from build123d import *

# Parameters (mm, degrees)
EXTRUDE_START   = 0.25
SKETCH_1_R      = 1.7
EXTRUDE_1_DEPTH = 6.5
SKETCH_2_R      = 5
SKETCH_2_R_2    = 1.7
EXTRUDE_2_DEPTH = 3


with BuildPart() as part:
    # 草图1 → 凸台-拉伸1 (new body)
    with BuildSketch(Plane.XY.offset(EXTRUDE_START)):
        with BuildLine():
            Line((198.226260921, 33.007621373), (206.908669804, -16.232766278))
            ThreePointArc((206.908669804, -16.232766278), (205.255667217, -20.882583864), (200.416253934, -21.848658507))
            Line((200.416253934, -21.848658507), (152.961109764, -6.171946743))
            ThreePointArc((152.961109764, -6.171946743), (148.598749605, -1.128713155), (150.97313978, 5.10239128))
            Line((150.97313978, 5.10239128), (190.204637372, 36.064296853))
            ThreePointArc((190.204637372, 36.064296853), (195.08261531, 36.811660465), (198.226260921, 33.007621373))
        make_face()
        with Locations((201.984631039, -17.101007166)):
            Circle(SKETCH_1_R, mode=Mode.SUBTRACT)
        with Locations((155, 0)):
            Circle(SKETCH_1_R, mode=Mode.SUBTRACT)
        with Locations((193.302222156, 32.139380484)):
            Circle(SKETCH_1_R, mode=Mode.SUBTRACT)
    extrude(amount=EXTRUDE_1_DEPTH)

    # 草图2 → 凸台-拉伸2 (add)
    with BuildSketch(Plane(origin=(0, 0, 0.25), x_dir=(-1, 0, 0), z_dir=(0, 0, -1))):
        with Locations((-201.984631039, -17.101007166)):
            Circle(SKETCH_2_R)
        with Locations((-201.984631039, -17.101007166)):
            Circle(SKETCH_2_R_2, mode=Mode.SUBTRACT)
    extrude(amount=EXTRUDE_2_DEPTH)


solid = part.part
The model under review builds one solid part; all positions refer to its coordinate system, in mm. Give positions to 0.01 mm unless a question says otherwise; leave off trailing zeros. Order: outer loops, then holes, each group sorted by start corner. A loop starts at its lowest first (then second) coordinate and runs counter-clockwise, first axis right, second up. Notation, with made-up numbers: M -35,-16 L 24,-16 A29 cw 24,17 Z; hole C -32,25 d10. An arc over 180 degrees is marked long. One line per question, with ' | ' between items. Start each with the question number.
1) Consider section C-C, the plane x = 155. Give the boundary of the cut face in (y, z).
2) Consider section B-B, the plane z = 1. Give the boundary of the cut face in (x, y).
3) Mouldability with a two-part tool opening along X and no side actions: class faces 1 (the face through (156.62, 0.51, 3.45)), 2 (the face through (148.616, -1.225, 3.454)), 3 (the face through (185, 8, 0.25)), 4 (the face through (194.873, 31.488, 3.454)) as pulls with the +X half, pulls with the -X half, needs draft (parallel to the pull), parting line crosses it, or undercut.
4) Wall thickness on L1, parallel to Z at x = 165, y = 0.5; L2, parallel to X at y = -2, z = 4; L3, parallel to X at y = 3, z = 1.75: over which ranges is each line inside the solid? List them lowest first. Write a range as from..to.
5) Consider section A-A, the plane y = 0. Give the boundary of the cut face in (x, z), then the cut area to 3 significant figures.
6) Clearance check with flat-ended pins moving along their axes: P1, Ø8, axis at x = 183, y = 22.5, coming from the -Z side; P2, Ø2, axis at y = 20.5, z = 0.5, coming from the -X side. State where each tip first meets the part, or that it passes through.
7) Consider section D-D, the plane x = 182. Give the boundary of the cut face in (y, z), then the cut area to 3 significant figures.
Found:
1) outline: M -6.85,0.25 L -1.7,0.25 L -1.7,6.75 L -6.85,6.75 Z; M 1.7,0.25 L 8.28,0.25 L 8.28,6.75 L 1.7,6.75 Z
2) outline: M 150.97,5.1 A6.5 ccw 152.96,-6.17 L 200.42,-21.85 A5 ccw 206.91,-16.23 L 198.23,33.01 A5 ccw 190.2,36.06 Z; hole C 155,0 d3.4; hole C 193.3,32.14 d3.4; hole C 201.98,-17.1 d3.4
3) face 1: undercut | face 2: pulls with the -X half | face 3: needs draft | face 4: undercut
4) L1: z = 0.25..6.75 | L2: x = 148.82..204.4 | L3: x = 149.23..203.52
5) outline: M 148.5,0.25 L 153.3,0.25 L 153.3,6.75 L 148.5,6.75 Z; M 156.7,0.25 L 204.05,0.25 L 204.05,6.75 L 156.7,6.75 Z | area: 339 mm²
6) P1: stops at z = 0.25 | P2: stops at x = 169.22
7) outline: M -15.76,0.25 L 29.59,0.25 L 29.59,6.75 L -15.76,6.75 Z | area: 295 mm²
